Geometry check sheet. Reference: drawing and pictorial views, mm from the part's lowest x, y, z. A direction names the side the tool comes from. Give positions to 0.01 mm unless a question says otherwise; leave off trailing zeros. Loops run counter-clockwise (first coordinate to the right, second up) from the corner with the lowest first, then second, coordinate; pieces in that order, holes last. Notation, with made-up numbers: M 2.25,-10.5 L 35.25,-10.5 A10 cw 35.25,0.5 Z; hole C 58.5,-26 d2. An arc over 180 degrees is marked long. Use CSV: the item, a comma, the result in double quotes.
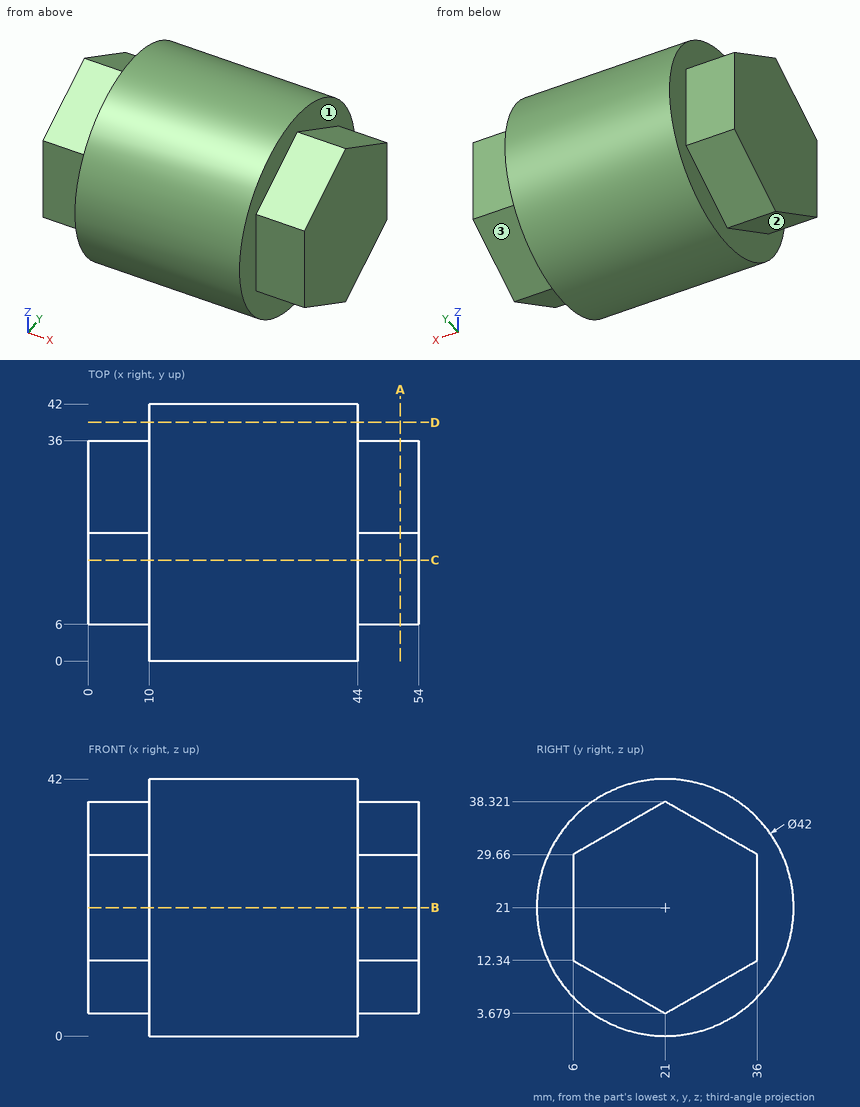
(1) Section check D-D on y = 39. Record the cut outline in (x, z).
Calculated:
outline,"M 10,10.18 L 44,10.18 L 44,31.82 L 10,31.82 Z"
(2) Tool access check on the marked faces 1, 2 and 3. Record the directions out of +Z, -Z, +X, -X, +Y, -Y that give a thin tool (end or side, any length) a straight path to the whole face; none if there is none.
Calculated:
face 1,"+X"
face 2,"-Z, -X, -Y"
face 3,"-Z, +X, +Y"
(3) Scan lines: L1, parallel to X at y = 12.5, z = 7; L2, parallel to Y at x = 5, z = 22; L3, parallel to Z at x = 29, y = 26.5. Record each from-to range of solid material in increasing order. Write a range as from..to.
Calculated:
L1,"x = 10..44"
L2,"y = 6..36"
L3,"z = 0.73..41.27"
(4) Section check A-A on x = 51. Record the cut outline in (y, z).
Calculated:
outline,"M 6,12.34 L 21,3.68 L 36,12.34 L 36,29.66 L 21,38.32 L 6,29.66 Z"
(5) Section check C-C on y = 16.5. Record the cut outline in (x, z), plus the area to 3 significant figures.
Calculated:
outline,"M 0,6.28 L 10,6.28 L 10,0.49 L 44,0.49 L 44,6.28 L 54,6.28 L 54,35.72 L 44,35.72 L 44,41.51 L 10,41.51 L 10,35.72 L 0,35.72 Z"
area,"1,980 mm²"
(6) Section check B-B on z = 21. Record the cut outline in (x, y), plus the area to 3 significant figures.
Calculated:
outline,"M 0,6 L 10,6 L 10,0 L 44,0 L 44,6 L 54,6 L 54,36 L 44,36 L 44,42 L 10,42 L 10,36 L 0,36 Z"
area,"2,030 mm²"
(7) Depth check by flat-ended pin: pin 1 Ø11 at (x, z) = (51, 19) entering from -Y; pin 2 Ø2 at (x, y) = (45.5, 23.5) entering from -Z (1 decimal); pin 3 Ø6 at (x, z) = (18.5, 5) entering from -Y. Enter the tip coordinate at first touch or a pass-through.
Calculated:
pin 1,"stops at y = 6"
pin 2,"stops at z = 4.5"
pin 3,"stops at y = 4.51"
